The drawing under review shows one solid part. Ordinate dimensions are in mm from its lowest x, y, z. Give positions to 0.01 mm unless a question says otherwise; leave off trailing zeros. Loops run counter-clockwise (first coordinate to the right, second up) from the corner with the lowest first, then second, coordinate; pieces in that order, holes last. Notation, with made-up numbers: M 53,53.25 L 73,53.25 A20 ccw 73,80.25 Z; hole C 79.25,72.25 d3. An arc over 180 degrees is marked long. One line per item, written item: value. Start each with the question number.
Q1. We need section C-C on y = 16.5. Write out the cut boundary in (x, z), plus the area to 4 significant figures.
Q2. To check wall thickness, follow line 1 along X through (y, z) = (34, 3) (3 decimals); line 2 along X through (y, z) = (19, 2) (3 decimals); line 3 along X through (y, z) = (13, 0.7). State the ranges of each line that lie inside material, in increasing order. Write a range as from..to.
Q3. We need section B-B on x = 130. Write out the cut boundary in (y, z).
Q4. We need section A-A on y = 32. Write out the cut boundary in (x, z) (3 decimals).
Q5. We need section D-D on y = 8.5. Write out the cut boundary in (x, z).
Q6. For pin 1 (1.8 mm diameter, centred on y = 7.5, z = 2, fed in from -X); pin 2 (2 mm diameter, centred on y = 8, z = 1, fed in from +X); pin 3 (1.8 mm diameter, centred on x = 90, z = 2, fed in from -Y), all flat-tipped, find the tip position at first contact; note any pin that passes through.
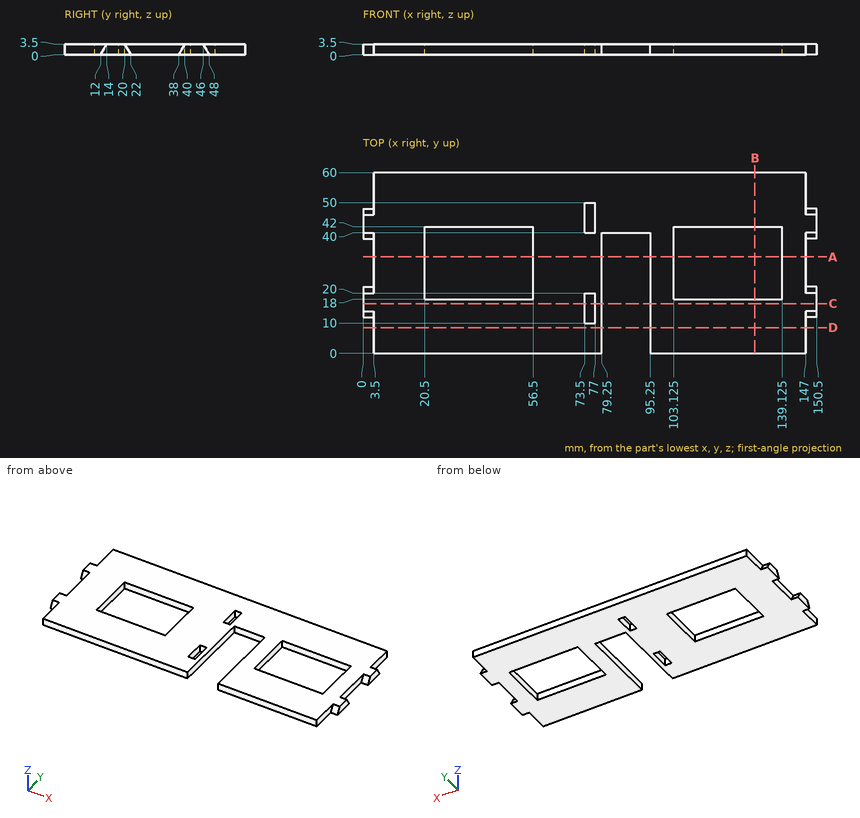
Solved:
1. outline: M 0,0 L 73.5,0 L 73.5,3.5 L 0,3.5 Z; M 77,0 L 79.25,0 L 79.25,3.5 L 77,3.5 Z; M 95.25,0 L 150.5,0 L 150.5,3.5 L 95.25,3.5 Z
1. area: 458.5 mm2
2. line 1: 3.5..20.5, 56.5..79.25, 95.25..103.125, 139.125..147
2. line 2: 0..20.5, 56.5..73.5, 77..79.25, 95.25..103.125, 139.125..150.5
2. line 3: 0..73.5, 77..79.25, 95.25..150.5
3. outline: M 0,0 L 18,0 L 18,3.5 L 0,3.5 Z; M 42,0 L 60,0 L 60,3.5 L 42,3.5 Z
4. outline: M 3.5,0 L 20.5,0 L 20.5,3.5 L 3.5,3.5 Z; M 56.5,0 L 79.25,0 L 79.25,3.5 L 56.5,3.5 Z; M 95.25,0 L 103.125,0 L 103.125,3.5 L 95.25,3.5 Z; M 139.125,0 L 147,0 L 147,3.5 L 139.125,3.5 Z
5. outline: M 3.5,0 L 79.25,0 L 79.25,3.5 L 3.5,3.5 Z; M 95.25,0 L 147,0 L 147,3.5 L 95.25,3.5 Z
6. pin 1: x = 3.5
6. pin 2: x = 147
6. pin 3: y = 40
